Read the model definition and answer for the solid it produces. Units are mm, in the model's axes. A direction names the side the tool comes from. Give positions to 0.01 mm unless a question says otherwise; leave off trailing zeros. Order: outer loops, then holes, each group sorted by start corner. A loop starts at its lowest first (then second) coordinate and runs counter-clockwise, first axis right, second up.
Item 1: Which of the six approach directions +Z, -Z, +X, -X, +Y, -Y give full straight-line access (tool end or side, diameter ignored) to faces 1 (the face through (45.82, 81.69, 39.13)), 2 (the face through (27.205, 77.114, 32.958)), 3 (the face through (76, 42, 36)), 4 (the face through (44.23, 5.393, 39.126))?
Item 2: A cutting plane is placed at D-D (x = 104.5). Write down the section's boundary in (y, z).
Item 3: A cutting plane is placed at B-B (z = 40). Write down the section's boundary in (x, y).
Item 4: A cutting plane is placed at A-A (x = 10). Write down the section's boundary in (y, z).
Item 5: A cutting plane is placed at C-C (y = 71). Write down the section's boundary in (x, z), plus the area to 3 significant figures.
Item 6: Given pin 1 Ø10 at (x, z) = (40, 31) entering from +Y; pin 2 Ø5.5 at (x, y) = (112, 44) entering from +Z; pin 3 Ø3.5 at (x, y) = (10, 45.01) entering from +Z; pin 4 Ø9.5 at (x, y) = (10, 80.02) entering from +Z, each flat-ended and moving along its own axis, determine where each tip first touches the part or whether it passes through.
Item 7: The mould has two halves that part along Z. Classify faces 5 (the face through (62, 80, 36)), 6 (the face through (12.77, 26.9, 32.96)), 7 (the face through (73.6, 79.8, 32.2)): +Z half, -Z half, draft (parallel to the pull), parting line (faces both ways), or undercut.
Item 8: Find the intervals of material crossed by line 1 along Y through (x, z) = (10, 28.75); line 2 along Z through (x, y) = (58.5, 10.5); line 3 along Y through (x, z) = (47, 38.25), in increasing order.
from build123d import *

# Parameters (mm, degrees)
SKETCH048_R                = 2.34
EXTRUDE050_DEPTH           = 20
SKETCH047_W                = 10
SKETCH047_H                = 20
EXTRUDE049_DEPTH           = 2
EXTRUDE049_PLACEMENT_ANGLE = 90
CUT121_PLACEMENT_ANGLE     = 96
CUT120_PLACEMENT_ANGLE     = 96
CUT119_PLACEMENT_ANGLE     = 84
CUT118_PLACEMENT_ANGLE     = 84
SKETCH018_R                = 1.955414
SKETCH018_R_2              = 1.945
SKETCH018_R_3              = 1.945712
EXTRUDE054_DEPTH           = 30
SKETCH017_R                = 2.552893
SKETCH017_R_2              = 2.443798
EXTRUDE192_DEPTH           = 7
SKETCH003_R                = 2.9
EXTRUDE052_DEPTH           = 50
EXTRUDE191_DEPTH           = 2


with BuildPart() as tornillos010:
    # Sketch048 (on Face6 of Extrude049) → Extrude050 (new body)
    with BuildSketch(Plane(origin=(-98, -107, 0), x_dir=(0, -1, 0), z_dir=(-1, 0, 0))):
        with Locations((-135.010223, 26.301971)):
            Circle(SKETCH048_R)
        with Locations((-135.047425, 15.116198)):
            Circle(SKETCH048_R)
    extrude(amount=EXTRUDE050_DEPTH)


with BuildPart() as tornillos010_1:
    # Extrude050 placement: moved
    add(tornillos010.part.moved(Location((17, 0, 0))))


with BuildPart() as soporte008:
    # Sketch047 → Extrude049 (new body)
    with BuildSketch(Plane.XZ):
        with Locations((-135, 20)):
            Rectangle(SKETCH047_W, SKETCH047_H)
    extrude(amount=EXTRUDE049_DEPTH)


with BuildPart() as soporte008_1:
    # Extrude049 placement: moved
    add(soporte008.part.moved(Location((-96, -107, 0))).rotate(Axis((-96, -107, 0), (0, 0, -1)), EXTRUDE049_PLACEMENT_ANGLE))


with BuildPart() as soporte024:
    # Cut121 base: copy of Soporte008
    add(soporte008_1.part)

    # Cut121: cut Tornillos010
    add(tornillos010_1.part, mode=Mode.SUBTRACT)


with BuildPart() as soporte024_1:
    # Cut121 placement: moved
    add(soporte024.part.moved(Location((7.869711, -10.850119, 18))).rotate(Axis((7.869711, -10.850119, 18), (0, 0, -1)), CUT121_PLACEMENT_ANGLE))


with BuildPart() as soporte023:
    # Cut120 base: copy of Soporte008
    add(soporte008_1.part)

    # Cut120: cut Tornillos010
    add(tornillos010_1.part, mode=Mode.SUBTRACT)


with BuildPart() as soporte023_1:
    # Cut120 placement: moved
    add(soporte023.part.moved(Location((37.705367, -13.985973, 18))).rotate(Axis((37.705367, -13.985973, 18), (0, 0, -1)), CUT120_PLACEMENT_ANGLE))


with BuildPart() as soporte022:
    # Cut119 base: copy of Soporte008
    add(soporte008_1.part)

    # Cut119: cut Tornillos010
    add(tornillos010_1.part, mode=Mode.SUBTRACT)


with BuildPart() as soporte022_1:
    # Cut119 placement: moved
    add(soporte022.part.moved(Location((26.348989, -93.015079, 18))).rotate(Axis((26.348989, -93.015079, 18), (0, 0, -1)), CUT119_PLACEMENT_ANGLE))


with BuildPart() as soporte021:
    # Cut118 base: copy of Soporte008
    add(soporte008_1.part)

    # Cut118: cut Tornillos010
    add(tornillos010_1.part, mode=Mode.SUBTRACT)


with BuildPart() as soporte021_1:
    # Cut118 placement: moved
    add(soporte021.part.moved(Location((77.069606, -87.684127, 18))).rotate(Axis((77.069606, -87.684127, 18), (0, 0, -1)), CUT118_PLACEMENT_ANGLE))


with BuildPart() as extrude054:
    # Sketch018 → Extrude054 (new body)
    with BuildSketch(Plane.XY.offset(36)):
        with Locations((74.789169, 44.062363)):
            Circle(SKETCH018_R)
        with Locations((111.023758, 44.110783)):
            Circle(SKETCH018_R)
        with Locations((29.159777, 78.682182)):
            Circle(SKETCH018_R_2)
        with Locations((60.039303, 78.850616)):
            Circle(SKETCH018_R_3)
        with Locations((64.412148, 25.488655)):
            Circle(SKETCH018_R_3)
    extrude(amount=EXTRUDE054_DEPTH)


with BuildPart() as extrude054_1:
    # Extrude054 placement: moved
    add(extrude054.part.moved(Location((0, 0, -22))))


with BuildPart() as base_tornillos001:
    # Sketch017 → Extrude192 (new body)
    with BuildSketch(Plane.XY.offset(30)):
        with Locations((74.792107, 44.0089)):
            Circle(SKETCH017_R)
        with Locations((111.059273, 44.092655)):
            Circle(SKETCH017_R)
        with Locations((60.050713, 78.85218)):
            Circle(SKETCH017_R_2)
        with Locations((29.144051, 78.600906)):
            Circle(SKETCH017_R_2)
        with Locations((14.570175, 25.247131)):
            Circle(SKETCH017_R_2)
        with Locations((64.40612, 25.414646)):
            Circle(SKETCH017_R_2)
    extrude(amount=EXTRUDE192_DEPTH)


with BuildPart() as base_tornillos001_1:
    # Extrude192 placement: moved
    add(base_tornillos001.part.moved(Location((0, 0, -1))))


with BuildPart() as tornillos053:
    # Sketch003 → Extrude052 (new body)
    with BuildSketch(Plane.XY.offset(10)):
        with Locations((10, 80.016689)):
            Circle(SKETCH003_R)
        with Locations((10, 45.008344)):
            Circle(SKETCH003_R)
        with Locations((10, 10)):
            Circle(SKETCH003_R)
    extrude(amount=EXTRUDE052_DEPTH)


with BuildPart() as tornillos053_1:
    # Extrude052 placement: moved
    add(tornillos053.part.moved(Location((0, 0, -21))))


with BuildPart() as obj1:
    # Sketch173 → Extrude191 (new body)
    with BuildSketch(Plane.XY):
        Polygon((0, 0), (30, 0), (120, 10), (120, 80), (30, 90), (0, 90), align=None)
    extrude(amount=EXTRUDE191_DEPTH)


with BuildPart() as obj1_1:
    # Extrude191 placement: moved
    add(obj1.part.moved(Location((0, 0, 28))))

    # Cut116: cut Tornillos053
    add(tornillos053_1.part, mode=Mode.SUBTRACT)

    # Fusion063: union Base tornillos001
    add(base_tornillos001_1.part)

    # Cut117: cut Extrude054
    add(extrude054_1.part, mode=Mode.SUBTRACT)

    # Fusion015: union Soporte021
    add(soporte021_1.part)

    # Fusion016: union Soporte022
    add(soporte022_1.part)

    # Fusion017: union Soporte023
    add(soporte023_1.part)

    # Fusion064: union Soporte024
    add(soporte024_1.part)


solid = obj1_1.part
Response values:
1. face 1: +Z, -X
1. face 2: +Z
1. face 3: +Z, +X, -X, -Y
1. face 4: +Z, +X, -Y
2. outline: (8.28, 28) - (81.72, 28) - (81.72, 30) - (8.28, 30) - close
3. outline: (38.98, 6.85) - (39.19, 4.86) - (49.13, 5.91) - (48.92, 7.9) - close; (40.78, 82.22) - (50.72, 81.17) - (50.93, 83.16) - (40.99, 84.21) - close; (70.61, 79.08) - (80.56, 78.04) - (80.77, 80.03) - (70.82, 81.07) - close; (89.7, 12.18) - (89.91, 10.19) - (99.85, 11.24) - (99.65, 13.23) - close
4. outline: (0, 28) - (7.1, 28) - (7.1, 30) - (0, 30) - close; (12.9, 28) - (42.11, 28) - (42.11, 30) - (12.9, 30) - close; (47.91, 28) - (77.12, 28) - (77.12, 30) - (47.91, 30) - close; (82.92, 28) - (90, 28) - (90, 30) - (82.92, 30) - close
5. outline: (0, 28) - (120, 28) - (120, 30) - (0, 30) - close
5. area: 240 mm2
6. pin 1: stops at y = 89.43
6. pin 2: stops at z = 36
6. pin 3: passes through
6. pin 4: stops at z = 30
7. face 5: +Z half
7. face 6: draft
7. face 7: undercut
8. line 1: y = 0 to 7.1, 12.9 to 42.11, 47.91 to 77.12, 82.92 to 90
8. line 2: z = 28 to 30
8. line 3: y = 5.68 to 7.7, 81.57 to 83.58
